```python
from build123d import *

# Parameters (mm, degrees)
F0_R      = 10.4
F0_R_2    = 8.8
F1_DEPTH  = 13.1
F2_DEPTH  = 25
F3_DEPTH  = 1.9
F4_R      = 10.9
F4_R_2    = 10.4
F5_DEPTH  = 17.7
F6_DEPTH  = 68.6
F7_R      = 10.9
F7_R_2    = 10.4
F7_R_3    = 8.8
F8_DEPTH  = 1
F9_R      = 10.4
F9_R_2    = 8.8
F10_DEPTH = 4
F11_R     = 10.9
F11_R_2   = 10.4
F11_R_3   = 8.8
F12_DEPTH = 10.3


with BuildPart() as f1:
    # F0 (on Right) → F1 (new body)
    with BuildSketch(Plane.YZ):
        Circle(F0_R)
        Circle(F0_R_2, mode=Mode.SUBTRACT)
        Circle(F0_R_2)
    extrude(amount=-F1_DEPTH)

    # F0 (on Right) → F2 (cut)
    with BuildSketch(Plane.YZ):
        Circle(F0_R_2)
    extrude(amount=-F2_DEPTH, mode=Mode.SUBTRACT)

    # F3 (add): a face of the model
    f3_faces = [f1.faces().sort_by_distance(p)[0] for p in [
        (-13.1, -10.105843579, 0),
    ]]
    extrude(f3_faces, amount=F3_DEPTH)

    # F4 (on face) + F0 (on Right) → F5 (join)
    with BuildSketch(Plane.YZ):
        Circle(F4_R)
        Circle(F4_R_2, mode=Mode.SUBTRACT)
    with BuildSketch(Plane.YZ):
        Circle(F0_R)
        Circle(F0_R_2, mode=Mode.SUBTRACT)
    extrude(amount=F5_DEPTH)

    # F0 (on Right) → F6 (join)
    with BuildSketch(Plane.YZ):
        Circle(F0_R)
        Circle(F0_R_2, mode=Mode.SUBTRACT)
    extrude(amount=F6_DEPTH)

    # F7 (on face) → F8 (join)
    with BuildSketch(Plane.YZ.offset(68.6)):
        Circle(F7_R)
        Circle(F7_R_2, mode=Mode.SUBTRACT)
        Circle(F7_R_2)
        Circle(F7_R_3, mode=Mode.SUBTRACT)
    extrude(amount=F8_DEPTH)

    # F9 (on face) → F10 (join)
    with BuildSketch(Plane.YZ.offset(69.6)):
        Circle(F9_R)
        Circle(F9_R_2, mode=Mode.SUBTRACT)
    extrude(amount=F10_DEPTH)

    # F11 (on face) → F12 (join)
    with BuildSketch(Plane.YZ.offset(73.6)):
        Circle(F11_R)
        Circle(F11_R_2, mode=Mode.SUBTRACT)
        Circle(F11_R_2)
        Circle(F11_R_3, mode=Mode.SUBTRACT)
    extrude(amount=F12_DEPTH)


solid = f1.part
```
Geometry: final body of the model. Coordinates: model frame, mm. A direction names the side the tool comes from. Round coordinates to 2 decimals unless told otherwise and drop trailing zeros. Loops run counter-clockwise (first coordinate to the right, second up) from the corner with the lowest first, then second, coordinate; pieces in that order, holes last. Notation, with made-up numbers: (27.5, 84.5) -> (85.5, 84.5) arc R5 cw to (85.5, 88.5) -> close; hole circle Ø11 at (-4.75, 25). An arc over 180 degrees is marked (long way). Use one line per item in the form item = value. Start each with the question number.
1) First-contact query: P1, Ø6, axis at x = 71, y = 3, coming from the -Z side; P2, Ø2, axis at y = -2.5, z = 7.5, coming from the -X side; P3, Ø2, axis at x = 17.5, z = -2.5, coming from the -Y side; P4, Ø4, axis at y = 0.5, z = 5, coming from the +X side. Flat tips, straight axial feed; report the tip coordinate or a pass-through.
2) Draft query along Y for faces 4 (the flat face through (83.9, 1, 9)), 5 (the cylindrical face through (71.57, -1.35, 10.31)), 6 (the cylindrical face through (33.758, 8.394, 2.643)). Return one class per face: released by +Y, released by -Y, zero draft, split by the parting line, or undercut.
3) Section A-A on y = 0. Output: boundary loops of the cut face in (x, z), then the cut area to 3 significant figures.
4) Section D-D on x = -5. Output: boundary loops of the cut face in (y, z), then the cut area to 3 significant figures.
5) Section C-C on x = 76. Output: boundary loops of the cut face in (y, z).
6) Access query for faces 1 (the flat face through (-15, -9, 2)), 2 (the cylindrical face through (42.79, -1.35, 10.31)), 3 (the cylindrical face through (-7.4, -1.35, 10.31)). Directions: +Z, -Z, +X, -X, +Y, -Y. A direction counts if a zero-diameter tool reaches every point of the face in a straight line with its end or side. Return the directions, or none.
7) Line query: L1, parallel to Z at x = 38.5, y = 0; L2, parallel to Z at x = 6, y = 0; L3, parallel to Y at x = 59.5, z = -1.5. Output: solid intervals per line, ascending.
Response:
q1.P1 = -10.89
q1.P2 = -15
q1.P3 = -10.8
q1.P4 = through
q2.face_4 = zero draft
q2.face_5 = split by the parting line
q2.face_6 = undercut
q3.outline = (-15, -10.4) -> (0, -10.4) -> (0, -10.9) -> (17.7, -10.9) -> (17.7, -10.4) -> (68.6, -10.4) -> (68.6, -10.9) -> (69.6, -10.9) -> (69.6, -10.4) -> (73.6, -10.4) -> (73.6, -10.9) -> (83.9, -10.9) -> (83.9, -8.8) -> (-15, -8.8) -> close; (-15, 8.8) -> (83.9, 8.8) -> (83.9, 10.9) -> (73.6, 10.9) -> (73.6, 10.4) -> (69.6, 10.4) -> (69.6, 10.9) -> (68.6, 10.9) -> (68.6, 10.4) -> (17.7, 10.4) -> (17.7, 10.9) -> (0, 10.9) -> (0, 10.4) -> (-15, 10.4) -> close
q3.area = 345 mm^2
q4.outline = circle Ø20.8 at (0, 0); hole circle Ø17.6 at (0, 0)
q4.area = 96.5 mm^2
q5.outline = circle Ø21.8 at (0, 0); hole circle Ø17.6 at (0, 0)
q6.face_1 = +Z, -Z, -X, +Y, -Y
q6.face_2 = none
q6.face_3 = -X
q7.L1 = -10.4 to -8.8, 8.8 to 10.4
q7.L2 = -10.9 to -8.8, 8.8 to 10.9
q7.L3 = -10.29 to -8.67, 8.67 to 10.29
